```python
from build123d import *

# Parameters (mm, degrees)
PAD_DEPTH       = 25
POCKET_DEPTH    = 25.001
SKETCH002_W     = 2
SKETCH002_H     = 4
POCKET001_DEPTH = 65.001


with BuildPart() as part:
    # Sketch → Pad (new body)
    with BuildSketch(Plane.XY):
        with BuildLine():
            Line((-15, 0), (-8.062258, 5))
            ThreePointArc((8.062258, 5), (0, 18), (-8.062258, 5))
            Line((8.062258, 5), (15, 0))
            Line((-15, 0), (15, 0))
        make_face()
    extrude(amount=PAD_DEPTH)

    # Sketch001 → Pocket (cut, through all)
    with BuildSketch(Plane.XY):
        with BuildLine():
            ThreePointArc((6.820042, 5.879579), (-6.596841, 12.568149), (6.344289, 5))
            Line((6.344289, 5), (8.062258, 5))
            ThreePointArc((8.062258, 5), (8.26371, 5.434737), (8.44174, 5.879579))
            Line((6.820042, 5.879579), (8.44174, 5.879579))
        make_face()
    extrude(amount=POCKET_DEPTH, mode=Mode.SUBTRACT)

    # Sketch002 → Pocket001 (cut, through all)
    with BuildSketch(Plane.YZ.offset(50)):
        with Locations((3, 21)):
            Rectangle(SKETCH002_W, SKETCH002_H)
        with Locations((3, 4)):
            Rectangle(SKETCH002_W, SKETCH002_H)
    extrude(amount=-POCKET001_DEPTH, mode=Mode.SUBTRACT)


solid = part.part
```
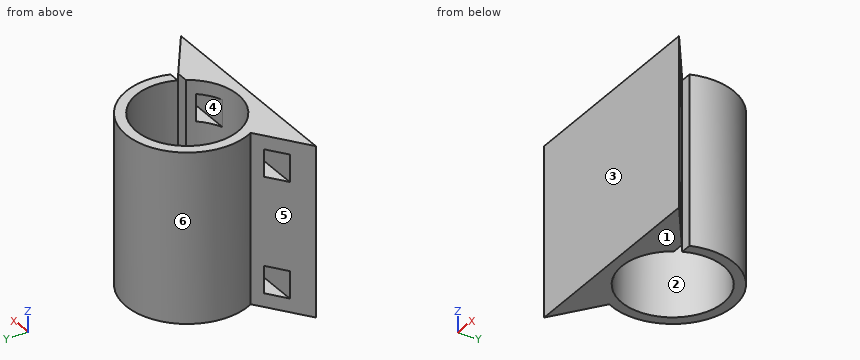
Here's how the part is built. I have some questions about the finished solid (model axes, mm). Face numbers are marked on the shaded views. A direction names the side the tool comes from. Round coordinates to 2 decimals unless told otherwise and drop trailing zeros. Order: outer loops, then holes, each group sorted by start corner. A loop starts at its lowest first (then second) coordinate and runs counter-clockwise, first axis right, second up. Notation, with made-up numbers: M -6,-24.75 L 3,-24.75 A23 cw 3,-5.75 Z; hole C 27.25,67.25 d4. An arc over 180 degrees is marked long. Answer in a Markdown table with one row per item.
Item 1: Imagine slicing it at A-A, the plane x = 0. Write out the boundary of the cut face in (y, z), and give its area (3 significant figures).
A:
| item | result |
|---|---|
| outline | M 0,0 L 1.5,0 L 1.5,25 L 0,25 Z; M 16.5,0 L 18,0 L 18,25 L 16.5,25 Z |
| area | 75.0 mm2 |
Item 2: For the marked faces 4, 5 and 6, which set-ups out of +Z, -Z, +X, -X, +Y, -Y let a thin tool reach every point of the face, with its end or its side?
A:
| item | result |
|---|---|
| face 4 | +X, -X |
| face 5 | +Z, -Z, -X |
| face 6 | +Z, -Z |
Item 3: Thinking about a two-plate mould opening in Y: for the marked faces 1, 2 and 3, which applies, +Y half, -Y half, draft (parallel to the pull), parting line (faces both ways), or undercut?
A:
| item | result |
|---|---|
| face 1 | draft |
| face 2 | undercut |
| face 3 | -Y half |
Item 4: If I drill on L1, parallel to Z at x = -9, y = 2.75; L2, parallel to Y at x = 0, z = 17.75; L3, parallel to Y at x = -6.5, z = 20.5, over which ranges is the centre line in solid material (lowest first)? Write a range as from..to.
A:
| item | result |
|---|---|
| L1 | z = 0..2, 6..19, 23..25 |
| L2 | y = 0..1.5, 16.5..18 |
| L3 | y = 0..2, 4..5.26, 12.74..15.22 |
Item 5: Imagine slicing it at C-C, the plane z = 21. Write out the boundary of the cut face in (x, y).
A:
| item | result |
|---|---|
| outline | M -15,0 L 15,0 L 12.22,2 L 2.69,2 A7.5 cw -2.69,2 L -12.22,2 Z; M -9.45,4 L -5.59,4 A7.5 cw long 6.82,5.88 L 8.44,5.88 A9 ccw long -8.06,5 Z; M 5.59,4 L 9.45,4 L 8.06,5 L 6.34,5 A7.5 cw Z |
Item 6: Imagine slicing it at B-B, the plane y = 9. Write out the boundary of the cut face in (x, z), and give its area (3 significant figures).
A:
| item | result |
|---|---|
| outline | M -9,0 L -7.5,0 L -7.5,25 L -9,25 Z; M 7.5,0 L 9,0 L 9,25 L 7.5,25 Z |
| area | 75.0 mm2 |
Item 7: Imagine slicing it at D-D, the plane x = -8.5. Write out the boundary of the cut face in (y, z), and give its area (3 significant figures).
A:
| item | result |
|---|---|
| outline | M 0,0 L 4.68,0 L 4.68,25 L 0,25 Z; M 6.04,0 L 11.96,0 L 11.96,25 L 6.04,25 Z; hole M 2,2 L 4,2 L 4,6 L 2,6 Z; hole M 2,19 L 4,19 L 4,23 L 2,23 Z |
| area | 249 mm2 |
Item 8: I'm going to push flat-ended pins straight in: pin 1 (6 mm diameter, centred on y = 14.5, z = 14.5, fed in from +X); pin 2 (1.2 mm diameter, centred on x = 8, z = 3.5, fed in from +Y); pin 3 (3 mm diameter, centred on x = -8, z = 3.5, fed in from +Y). Where does each tip first touch, or does it pass through?
A:
| item | result |
|---|---|
| pin 1 | stops at x = 8.65 |
| pin 2 | stops at y = 14.12 |
| pin 3 | stops at y = 15.22 |
